Could you check a few things on this model? Use its own coordinates, in mm. Face numbers are marked on the shaded views. A direction names the side the tool comes from. Coordinates: 2 decimals unless noted, no trailing zeros. Write each loop counter-clockwise with the first axis right and the second up, starting at its lowest first coordinate (ties: lowest second). Pieces come first, ordered by that corner, then holes. Notation, with made-up numbers: (22.5, 21) - (44.5, 21) arc R29 ccw to (44.5, 47) - close; hole circle Ø7 at (43.25, 36.25). An arc over 180 degrees is marked (long way). Answer as a JSON object with one key per item and string values. Group by question number.
1) On a 3-axis mill with a long thin cutter (end or side, diameter ignored), from which of +Z, -Z, +X, -X, +Y, -Y can I reach the whole of each face in a straight line? I mean the marked faces 1 and 2. Say none if no direction works.
2) We'd pull the mould along Z, two halves only. Please class the marked faces 3, 4 and 5: released by +Z, released by -Z, zero draft, split by the parting line, or undercut.
3) If we section it at A-A (y = -18.5): Write out the boundary of the cut face in (x, z).
4) If we section it at C-C (y = 3): Write out the boundary of the cut face in (x, z), plus the area to 3 significant figures.
5) Will these pins go through, and if not, where does the flat tip stop? pin 1 Ø1.5 at (x, y) = (-3.5, -2) entering from +Z; pin 2 Ø4 at (x, y) = (-5, -6.5) entering from +Z; pin 3 Ø1 at (x, y) = (5.5, 10) entering from +Z; pin 4 Ø7.5 at (x, z) = (0, 0) entering from -Y.
6) If we section it at B-B (z = -5): Write out the boundary of the cut face in (x, y), plus the area to 3 significant figures.
7) Please list where these lines run through material, in increasing order: line 1 along Z through (x, y) = (-0.25, 10.5); line 2 along X through (y, z) = (-17.5, -3).
Autodesk Inventor part; units mm, degrees
ref_plane "YZ Plane" through (0, 0, 0) normal (1, 0, 0) x (0, 1, 0)
ref_plane "XZ Plane" through (0, 0, 0) normal (0, 1, 0) x (-1, 0, 0)
ref_plane "XY Plane" through (0, 0, 0) normal (0, 0, 1) x (1, 0, 0)
sketch "Sketch1" plane through (0, 0, 0) normal (0, 1, 0) x (-1, 0, 0)
  circle A0 centre (0, 0) radius 7.5
  dimension "d0" = 15
extrude "Extrusion1" add sketch "Sketch1" along normal mid plane 49
sketch "Sketch2" plane through (0, 24.5, 0) normal (0, 1, 0) x (1, 0, 0)
  point P0 (0, 0)
  point P1 (0, 0)
hole "Hole1" at (0, 24.5, 0) direction (0, -1, 0) diameter 6.647 depth 20 tip angle 118
mirror "Mirror2" about plane through (0, 0, 0) normal (0, 1, 0) of "Hole1"
properties part number "Mid_structure_bar"
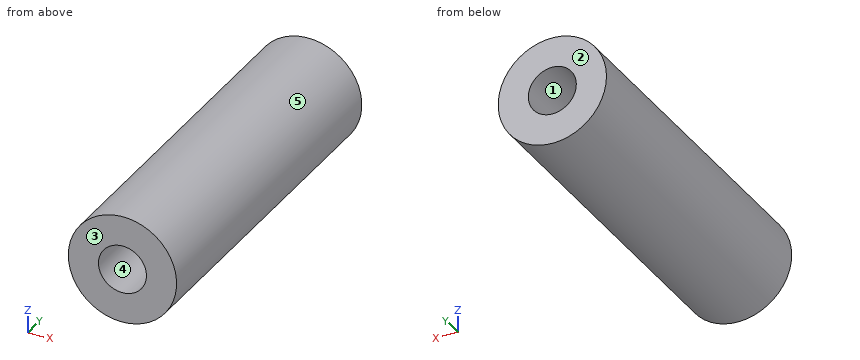
Here are the results:
{
 "1": {"face 1": "+Y", "face 2": "+Z, -Z, +X, -X, +Y"},
 "2": {"face 3": "zero draft", "face 4": "undercut", "face 5": "split by the parting line"},
 "3": {"outline": "circle Ø15 at (0, 0); hole circle Ø6.65 at (0, 0)"},
 "4": {"outline": "circle Ø15 at (0, 0); hole circle Ø1.65 at (0, 0)", "area": "175 mm²"},
 "5": {"pin 1": "stops at z = 6.98", "pin 2": "stops at z = 6.87", "pin 3": "stops at z = 5.59", "pin 4": "stops at y = -24.5"},
 "6": {"outline": "(-5.59, -24.5) - (5.59, -24.5) - (5.59, 24.5) - (-5.59, 24.5) - close", "area": "548 mm²"},
 "7": {"line 1": "z = -7.5 to -3.31, 3.31 to 7.5", "line 2": "x = -6.87 to -1.43, 1.43 to 6.87"}
}
